Input: part model. Units: mm. Frame: model coordinates. Face numbers are marked on the shaded views. A direction names the side the tool comes from. Round coordinates to 2 decimals unless told otherwise and drop trailing zeros. Loops run counter-clockwise (first coordinate to the right, second up) from the corner with the lowest first, then second, coordinate; pieces in that order, holes last. Notation, with made-up numbers: (42, 25.25) - (53, 25.25) arc R25 ccw to (53, 59.25) - close; hole circle Ø6 at (10.5, 74.25). An arc over 180 degrees is marked (long way). One line per question, with ' | ' between items. Start each with the question number.
Item 1: Material intervals for line 1 along Y through (x, z) = (-17.5, -5.4); line 2 along Z through (x, y) = (9, 4.25); line 3 along Z through (x, y) = (-6.5, -6), sorted ascending.
Item 2: Section A-A, the plane y = 0. Give the number of separate pieces and of enclosed holes in the cut face, plus the area to 3 significant figures.
Item 3: First-contact query: pin 1 (6 mm diameter, centred on x = -21, z = -2, fed in from -Y); pin 2 (1.5 mm diameter, centred on x = -19.5, z = 5, fed in from -Y); pin 3 (5.5 mm diameter, centred on x = -16.5, y = -1, fed in from -Z); pin 4 (4 mm diameter, centred on x = -17.5, y = 0, fed in from +Z). Flat tips, straight axial feed; report the tip coordinate or a pass-through.
Item 4: Section C-C, the plane z = 5.5. Return loops of the section in (x, y).
Item 5: Section D-D, the plane x = 9.5. Return loops of the section in (y, z).
Item 6: Section B-B, the plane x = -12. Return loops of the section in (y, z).
Item 7: Draft query along X for the marked faces 4, 5, 6 and 7. Return one class per face: pulls with the +X half, pulls with the -X half, needs draft (parallel to the pull), parting line crosses it, or undercut.
Item 8: Set-up query: the marked faces 1, 2 and 3. Return all of +Z, -Z, +X, -X, +Y, -Y with unobstructed straight access to the full face (end or side cutting, diameter ignored); none if empty.
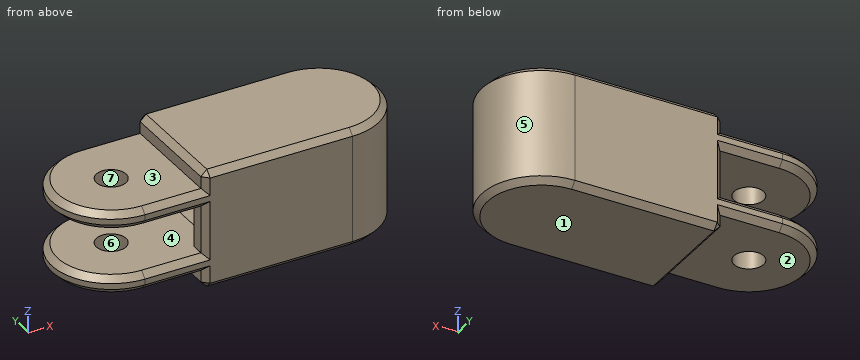
```python
from build123d import *

# Parameters (mm, degrees)
BOSS_EXTRUDE1_DEPTH = 10
CUT_EXTRUDE1_DEPTH  = 4
CUT_EXTRUDE2_START  = -7
CUT_EXTRUDE2_DEPTH  = 7
CUT_EXTRUDE3_START  = 14
CUT_EXTRUDE3_DEPTH  = 7
SKETCH3_R           = 2.5
CUT_EXTRUDE4_DEPTH  = 10
SHELL1_START        = -7
SHELL1_DEPTH        = 14
SHELL1_START_2      = -4
SHELL1_2_OUTLINE_W  = 3
SHELL1_2_OUTLINE_H  = 14
SHELL1_2_DEPTH      = 8
CHAMFER1_SIZE       = 1


# Read off the part's stored shape, not the designer's step: Shell1
with BuildPart() as part:
    # Sketch1 → Boss-Extrude1 (new, symmetric)
    with BuildSketch(Plane.XY):
        with BuildLine():
            Line((-17.5, 10), (17.5, 10))
            ThreePointArc((17.5, 10), (27.5, 0), (17.5, -10))
            Line((17.5, -10), (-17.5, -10))
            ThreePointArc((-17.5, -10), (-27.5, 0), (-17.5, 10))
        make_face()
    extrude(amount=BOSS_EXTRUDE1_DEPTH, both=True)

    # Sketch2 → Cut-Extrude1 (cut, symmetric)
    with BuildSketch(Plane.XY):
        with BuildLine():
            Line((-17.5, 10), (-7.5, 10))
            Line((-7.5, 10), (-7.5, -10))
            Line((-7.5, -10), (-17.5, -10))
            ThreePointArc((-17.5, -10), (-27.5, 0), (-17.5, 10))
        make_face()
    extrude(amount=CUT_EXTRUDE1_DEPTH, both=True, mode=Mode.SUBTRACT)

    # Sketch2<2> → Cut-Extrude2 (cut)
    with BuildSketch(Plane.XY.offset(CUT_EXTRUDE2_START)):
        with BuildLine():
            Line((-17.5, 10), (-7.5, 10))
            Line((-7.5, 10), (-7.5, -10))
            Line((-7.5, -10), (-17.5, -10))
            ThreePointArc((-17.5, -10), (-27.5, 0), (-17.5, 10))
        make_face()
    extrude(amount=-CUT_EXTRUDE2_DEPTH, mode=Mode.SUBTRACT)

    # Sketch2<3> → Cut-Extrude3 (cut)
    with BuildSketch(Plane.XY.offset(CUT_EXTRUDE3_START)):
        with BuildLine():
            Line((-17.5, 10), (-7.5, 10))
            Line((-7.5, 10), (-7.5, -10))
            Line((-7.5, -10), (-17.5, -10))
            ThreePointArc((-17.5, -10), (-27.5, 0), (-17.5, 10))
        make_face()
    extrude(amount=-CUT_EXTRUDE3_DEPTH, mode=Mode.SUBTRACT)

    # Sketch3 → Cut-Extrude4 (cut, symmetric)
    with BuildSketch(Plane.XY):
        with Locations((-17.5, 0)):
            Circle(SKETCH3_R)
    extrude(amount=CUT_EXTRUDE4_DEPTH, both=True, mode=Mode.SUBTRACT)

    # Shell1 outline → Shell1 (cut)
    with BuildSketch(Plane.XY.offset(SHELL1_START)):
        with BuildLine():
            Line((-4.5, -7), (17.5, -7))
            ThreePointArc((17.5, -7), (24.5, 0), (17.5, 7))
            Line((17.5, 7), (-4.5, 7))
            Line((-4.5, 7), (-4.5, -7))
        make_face()
    extrude(amount=SHELL1_DEPTH, mode=Mode.SUBTRACT)

    # Shell1 2 outline → Shell1 2 (cut)
    with BuildSketch(Plane.XY.offset(SHELL1_START_2)):
        with Locations((-6, 0)):
            Rectangle(SHELL1_2_OUTLINE_W, SHELL1_2_OUTLINE_H)
    extrude(amount=SHELL1_2_DEPTH, mode=Mode.SUBTRACT)

    # Chamfer1
    chamfer1_edges = [part.edges().sort_by_distance(p)[0] for p in [
        (27.5, 0, 10),
        (5, 10, 10),
        (-27.5, 0, -4),
        (-12.5, 10, -4),
        (-7.5, 10, 0),
        (-12.5, -10, -4),
        (-7.5, -10, 0),
        (-27.5, 0, 4),
        (-12.5, -10, 4),
        (-12.5, 10, 4),
        (5, -10, -10),
        (-7.5, 0, -10),
        (-7.5, 10, -8.5),
        (-7.5, -10, -8.5),
        (-27.5, 0, -7),
        (-12.5, -10, -7),
        (-12.5, 10, -7),
        (5, 10, -10),
        (5, -10, 10),
        (-7.5, 0, 10),
        (27.5, 0, -10),
        (-27.5, 0, 7),
        (-12.5, -10, 7),
        (-7.5, -10, 8.5),
        (-7.5, 10, 8.5),
        (-12.5, 10, 7),
    ]]
    chamfer(chamfer1_edges, length=CHAMFER1_SIZE)


solid = part.part
```
Return value:
1) line 1: -10 to -2.5, 2.5 to 10 | line 2: -10 to -7, 7 to 10 | line 3: -10 to -4, 4 to 10
2) separate pieces: 3 | enclosed holes: 0 | area: 356 mm2
3) pin 1: y = -9.52 | pin 2: y = -9.92 | pin 3: z = -7 | pin 4: through
4) outline: (-17.5, -10) - (17.5, -10) arc R10 ccw to (17.5, 10) - (-17.5, 10) arc R10 ccw to start; hole circle Ø5 at (-17.5, 0); hole (-4.5, -7) - (17.5, -7) arc R7 ccw to (17.5, 7) - (-4.5, 7) - close
5) outline: (-10, -9) - (-9, -10) - (9, -10) - (10, -9) - (10, 9) - (9, 10) - (-9, 10) - (-10, 9) - close; hole (-7, -7) - (7, -7) - (7, 7) - (-7, 7) - close
6) outline: (-10, -6) - (-9, -7) - (9, -7) - (10, -6) - (10, -5) - (9, -4) - (-9, -4) - (-10, -5) - close; (-10, 5) - (-9, 4) - (9, 4) - (10, 5) - (10, 6) - (9, 7) - (-9, 7) - (-10, 6) - close
7) face 4: needs draft | face 5: pulls with the +X half | face 6: undercut | face 7: undercut
8) face 1: -Z, +X, -X, +Y, -Y | face 2: -Z, -X, +Y, -Y | face 3: +Z, -X, +Y, -Y
